Verification items for the finished model (mm, model axes). Face numbers are marked on the shaded views. A direction names the side the tool comes from. Coordinates: 2 decimals unless noted, no trailing zeros. Loops run counter-clockwise (first coordinate to the right, second up) from the corner with the lowest first, then second, coordinate; pieces in that order, holes last. Notation, with made-up numbers: (11.5, -38.5) -> (19.5, -38.5) arc R26 ccw to (19.5, 0.5) -> close; hole circle Ø10 at (50, 15.5). An arc over 180 degrees is marked (long way). Answer as a JSON object with one key per item and string values. Group by question number.
Q1. Cross-section at D-D on y = -11.5. Give the number of separate pieces and of enclosed holes in the cut face, and give its area (3 significant figures).
Q2. Cross-section at A-A on y = 19. Record the boundary of the cut face in (x, z) (3 decimals).
Q3. Set-up check for the marked faces 5, 6 and 7: record each of +Z, -Z, +X, -X, +Y, -Y from which the full face is reachable in a straight line by a thin tool's end or side.
Q4. Release check for a two-part mould opening along X. For the marked faces 1, 2, 3 and 4 record: released by +X, released by -X, zero draft, split by the parting line, or undercut.
Q5. Gauge pin test, flat ends, axial feed: pin 1 Ø1.9 at (x, y) = (6.35, 15.875) entering from +Z; pin 2 Ø3 at (x, z) = (7.5, 0.5) entering from +Y (3 decimals). Record the tip position at first contact, or that the pin passes through.
Q6. Cross-section at B-B on x = -7. Record the boundary of the cut face in (y, z) (3 decimals), and give its area (3 significant figures).
Q7. Scan lines: L1, parallel to Y at x = 16.25, z = 0 (3 decimals); L2, parallel to Z at x = 13.5, y = 5 (3 decimals); L3, parallel to X at y = 10.5, z = -0.25. Record each from-to range of solid material in increasing order.
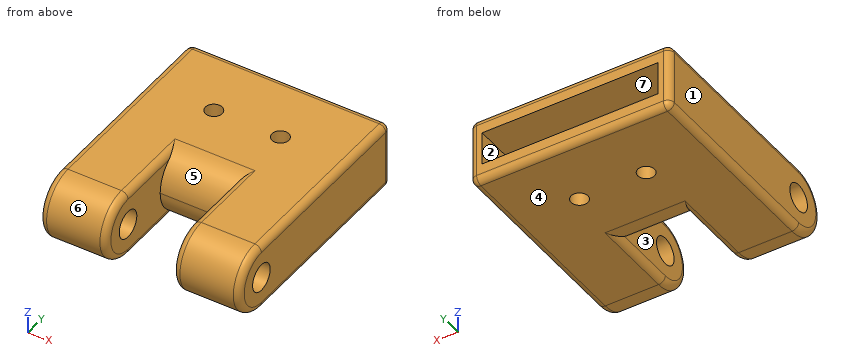
```python
from build123d import *

# Parameters (mm, degrees)
ESQUISSE1_W             = 38.1
ESQUISSE1_H             = 12.7
BOSS_EXTRU_1_DEPTH      = 3.175
ESQUISSE2_W             = 38.1
ESQUISSE2_H             = 12.7
ESQUISSE2_W_2           = 33.4518
ESQUISSE2_H_2           = 6.35
BOSS_EXTRU_2_DEPTH      = 25.4
ESQUISSE3_R             = 1.6
ENL_V_MAT_EXTRU_1_DEPTH = 25.4
ESQUISSE4_R             = 2.6
BOSS_EXTRU_3_DEPTH      = 12.7
CONG_1_R                = 6.35
CONG_2_R                = 1.27


with BuildPart() as part:
    # Esquisse1 → Boss.-Extru.1 (new body)
    with BuildSketch(Plane(origin=(0, 0, 0), x_dir=(1, 0, 0), z_dir=(0, 1, 0))):
        Rectangle(ESQUISSE1_W, ESQUISSE1_H)
    extrude(amount=BOSS_EXTRU_1_DEPTH)

    # Esquisse2 → Boss.-Extru.2 (add)
    with BuildSketch(Plane(origin=(0, 3.175, 0), x_dir=(1, 0, 0), z_dir=(0, 1, 0))):
        Rectangle(ESQUISSE2_W, ESQUISSE2_H)
        Rectangle(ESQUISSE2_W_2, ESQUISSE2_H_2, mode=Mode.SUBTRACT)
    extrude(amount=BOSS_EXTRU_2_DEPTH)

    # Esquisse3 → Enlèv. mat.-Extru.1 (cut)
    with BuildSketch(Plane.XY.offset(6.35)):
        with Locations((-6.35, 15.875)):
            Circle(ESQUISSE3_R)
        with Locations((6.35, 15.875)):
            Circle(ESQUISSE3_R)
    extrude(amount=-ENL_V_MAT_EXTRU_1_DEPTH, mode=Mode.SUBTRACT)

    # Esquisse4 → Boss.-Extru.3 (add)
    with BuildSketch(Plane(origin=(19.05, 0, 0), x_dir=(0, 0, -1), z_dir=(1, 0, 0))):
        with BuildLine():
            Line((-6.35, 0), (-6.35, -9.525))
            ThreePointArc((-6.35, -9.525), (0, -15.875), (6.35, -9.525))
            Line((6.35, -9.525), (6.35, 0))
            Line((6.35, 0), (-6.35, 0))
        make_face()
        with Locations((0, -9.525)):
            Circle(ESQUISSE4_R, mode=Mode.SUBTRACT)
    boss_extru_3 = extrude(amount=-BOSS_EXTRU_3_DEPTH)

    # Symétrie1: Boss.-Extru.3 across plane
    add(boss_extru_3.mirror(Plane(origin=(0, 0, 0), x_dir=(0, 0, 1), z_dir=(1, 0, 0))))

    # Congé1
    cong_1_edges = [part.edges().sort_by_distance(p)[0] for p in [
        (0, 0, -6.35),
        (0, 0, 6.35),
    ]]
    fillet(cong_1_edges, radius=CONG_1_R - 0.0001)  # a hair under: the kernel refuses the full size

    # Congé2
    cong_2_edges = [part.edges().sort_by_distance(p)[0] for p in [
        (-19.05, 28.575, 0),
        (0, 28.575, 6.35),
        (19.05, 28.575, 0),
        (0, 28.575, -6.35),
        (6.35, -1.58755, -6.35),
        (6.35, -15.875, 0),
        (6.35, -1.58755, 6.35),
        (19.05, -15.875, 0),
        (-6.35, -1.58755, 6.35),
        (-6.35, -15.875, 0),
        (-6.35, -1.58755, -6.35),
        (-19.05, -15.875, 0),
        (19.05, 9.525, 6.35),
        (-19.05, 9.525, 6.35),
        (-19.05, 9.525, -6.35),
        (19.05, 9.525, -6.35),
    ]]
    fillet(cong_2_edges, radius=CONG_2_R)


solid = part.part
```
Computed values:
{
 "1": {"separate pieces": "4", "enclosed holes": "0", "area": "218 mm²"},
 "2": {"outline": "(-19.05, -5.08) arc R1.27 ccw to (-17.78, -6.35) -> (17.78, -6.35) arc R1.27 ccw to (19.05, -5.08) -> (19.05, 5.08) arc R1.27 ccw to (17.78, 6.35) -> (-17.78, 6.35) arc R1.27 ccw to (-19.05, 5.08) -> close; hole (-16.726, -3.175) -> (16.726, -3.175) -> (16.726, 3.175) -> (-16.726, 3.175) -> close"},
 "3": {"face 5": "+Z, -Y", "face 6": "+X, -X, -Y", "face 7": "+Y"},
 "4": {"face 1": "released by -X", "face 2": "undercut", "face 3": "undercut", "face 4": "zero draft"},
 "5": {"pin 1": "passes through", "pin 2": "stops at y = 3.175"},
 "6": {"outline": "(-9.525, -6.188) -> (4.926, -6.188) arc R6.35 ccw to (6.35, -6.35) -> (14.413, -6.35) -> (14.413, -3.175) -> (3.175, -3.175) -> (3.175, 3.175) -> (14.413, 3.175) -> (14.413, 6.35) -> (6.35, 6.35) arc R6.35 ccw to (4.926, 6.188) -> (-9.525, 6.188) arc R6.188 ccw to start; (17.337, -6.35) -> (27.305, -6.35) arc R1.27 ccw to (28.575, -5.08) -> (28.575, -3.175) -> (17.337, -3.175) -> close; (17.337, 3.175) -> (28.575, 3.175) -> (28.575, 5.08) arc R1.27 ccw to (27.305, 6.35) -> (17.337, 6.35) -> close; hole circle Ø5.2 at (-9.525, 0)", "area": "337 mm²"},
 "7": {"L1": "y = -15.875 to -12.125, -6.925 to 3.175", "L2": "z = -6.35 to -3.175, 3.175 to 6.35", "L3": "x = -19.05 to -16.73, 16.73 to 19.05"}
}
